Build history of the part. All positions in model axes, mm. Face numbers are marked on the shaded views. A direction names the side the tool comes from. Coordinates: 2 decimals unless noted, no trailing zeros. Order: outer loops, then holes, each group sorted by start corner. A loop starts at its lowest first (then second) coordinate and runs counter-clockwise, first axis right, second up. Notation, with made-up numbers: (-38, -17.75) - (-19, -17.75) arc R23 cw to (-19, 8.25) - close; hole circle Ø3 at (-29.75, 76.5). An arc over 180 degrees is marked (long way). One line per item, written item: value.
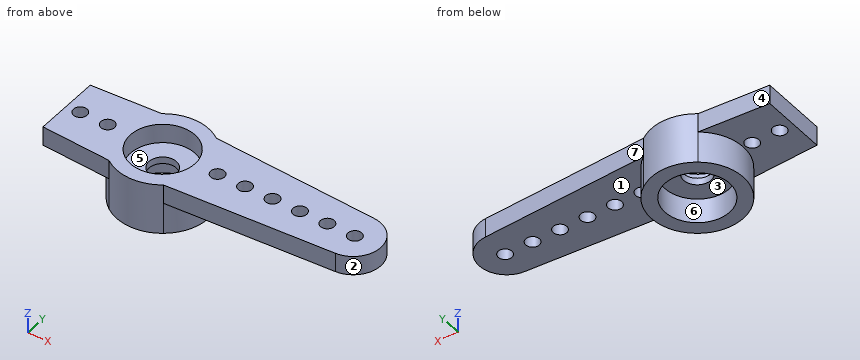
from build123d import *

# Parameters (mm, degrees)
F0_R     = 2.35
F0_R_2   = 0.5
F1_DEPTH = 1.4
F2_R     = 2.35
F2_R_2   = 1
F3_DEPTH = 2.3
F4_R     = 2.35
F4_R_2   = 1
F5_DEPTH = 1.8


with BuildPart() as f1:
    # F0 (on Top) → F1 (new body)
    with BuildSketch(Plane.XY):
        with BuildLine():
            ThreePointArc((1.9830532015, -2.7), (2.9887897404, -1.5131542841), (3.35, 0))
            ThreePointArc((3.35, 0), (2.9887897404, 1.5131542841), (1.9830532015, 2.7))
            ThreePointArc((1.9830532015, 2.7), (0, 3.35), (-1.9830532015, 2.7))
            ThreePointArc((-1.9830532015, 2.7), (-3.35, 0), (-1.9830532015, -2.7))
            ThreePointArc((-1.9830532015, -2.7), (0, -3.35), (1.9830532015, -2.7))
        make_face()
        Circle(F0_R, mode=Mode.SUBTRACT)
        with BuildLine():
            ThreePointArc((1.9830532015, 2.7), (2.9887897404, 1.5131542841), (3.35, 0))
            ThreePointArc((3.35, 0), (2.9887897404, -1.5131542841), (1.9830532015, -2.7))
            Line((1.9830532015, -2.7), (14, -2))
            ThreePointArc((14, -2), (15.886888175, 0), (14, 2))
            Line((14, 2), (1.9830532015, 2.7))
        make_face()
        with Locations((4, 0)):
            Circle(F0_R_2, mode=Mode.SUBTRACT)
        with Locations((6, 0)):
            Circle(F0_R_2, mode=Mode.SUBTRACT)
        with Locations((8, 0)):
            Circle(F0_R_2, mode=Mode.SUBTRACT)
        with Locations((10, 0)):
            Circle(F0_R_2, mode=Mode.SUBTRACT)
        with Locations((12, 0)):
            Circle(F0_R_2, mode=Mode.SUBTRACT)
        with Locations((14, 0)):
            Circle(F0_R_2, mode=Mode.SUBTRACT)
        with BuildLine():
            ThreePointArc((-1.9830532015, -2.7), (-3.35, 0), (-1.9830532015, 2.7))
            Line((-1.9830532015, 2.7), (-6.9970610693, 2.4079286805))
            Line((-6.9970610693, 2.4079286805), (-6.9970610693, -2.4079286805))
            Line((-6.9970610693, -2.4079286805), (-1.9830532015, -2.7))
        make_face()
        with Locations((-6, 0)):
            Circle(F0_R_2, mode=Mode.SUBTRACT)
        with Locations((-4, 0)):
            Circle(F0_R_2, mode=Mode.SUBTRACT)
    extrude(amount=F1_DEPTH)

    # F2 (on face) → F3 (join)
    with BuildSketch(Plane(origin=(0, 0, 0), x_dir=(1, 0, 0), z_dir=(0, 0, -1))):
        with BuildLine():
            ThreePointArc((1.9830532015, -2.7), (2.9887897404, -1.5131542841), (3.35, 0))
            ThreePointArc((3.35, 0), (2.9887897404, 1.5131542841), (1.9830532015, 2.7))
            ThreePointArc((1.9830532015, 2.7), (0, 3.35), (-1.9830532015, 2.7))
            ThreePointArc((-1.9830532015, 2.7), (-3.35, 0), (-1.9830532015, -2.7))
            ThreePointArc((-1.9830532015, -2.7), (0, -3.35), (1.9830532015, -2.7))
        make_face()
        Circle(F2_R, mode=Mode.SUBTRACT)
        Circle(F2_R)
        Circle(F2_R_2, mode=Mode.SUBTRACT)
    extrude(amount=F3_DEPTH)

    # F4 (on face) → F5 (cut)
    with BuildSketch(Plane(origin=(0, 0, -2.3), x_dir=(1, 0, 0), z_dir=(0, 0, -1))):
        Circle(F4_R)
        Circle(F4_R_2, mode=Mode.SUBTRACT)
    extrude(amount=-F5_DEPTH, mode=Mode.SUBTRACT)


solid = f1.part
1. 3-axis set-ups, long thin cutter, end or side, ignore diameter. For the marked faces 5, 6 and 7: which of +Z, -Z, +X, -X, +Y, -Y reach the whole face in a straight line?
Values found:
face 5: +Z
face 6: -Z
face 7: +Z, -Z, +X, +Y
2. Band-saw the part on A-A, the plane z = 0.35. Count the separate pieces of the cut face and the enclosed holes in it, and give its area (3 significant figures).
Values found:
separate pieces: 1
enclosed holes: 9
area: 89.2 mm2
3. Probe line 1 along Y through (x, z) = (8, 0.7); line 2 along X through (y, z) = (0, -1.5); line 3 along Z through (x, y) = (-3.5, -1.5). List the from-to ranges inside material, lowest first.
Values found:
line 1: y = -2.35 to -0.5, 0.5 to 2.35
line 2: x = -3.35 to -2.35, 2.35 to 3.35
line 3: z = 0 to 1.4
4. Band-saw the part on C-C, the plane y = 1.5. Give the cut face in (x, z).
Values found:
outline: (-7, 0) - (-3, 0) - (-3, -2.3) - (-1.81, -2.3) - (-1.81, -0.5) - (1.81, -0.5) - (1.81, -2.3) - (3, -2.3) - (3, 0) - (15.21, 0) - (15.21, 1.4) - (1.81, 1.4) - (1.81, 0) - (-1.81, 0) - (-1.81, 1.4) - (-7, 1.4) - close
5. Band-saw the part on B-B, the plane x = 12. Give the cut face in (y, z), and give its area (3 significant figures).
Values found:
outline: (-2.12, 0) - (-0.5, 0) - (-0.5, 1.4) - (-2.12, 1.4) - close; (0.5, 0) - (2.12, 0) - (2.12, 1.4) - (0.5, 1.4) - close
area: 4.53 mm2
6. Band-saw the part on D-D, the plane z = -1.55. Give the cut face in (x, y).
Values found:
outline: circle Ø6.7 at (0, 0); hole circle Ø4.7 at (0, 0)
7. Flat gauge pins, fed straight in: P1, Ø1.6, axis at x = 7.5, y = 1, coming from the -Z side; P2, Ø1.4, axis at x = -1, y = -0.5, coming from the +Z side; P3, Ø1.5, axis at y = -1.5, z = -1, coming from the +X side; P4, Ø1.6, axis at x = 0, y = 0, coming from the -Z side. Where does each tip first touch, or does it go through?
Values found:
P1: stops at z = 0
P2: stops at z = 0
P3: stops at x = 3.26
P4: passes through
8. Two-plate mould, pull along Y, no slides. Class the marked faces 1, 2, 3 and 4: pulls with the +Y half, pulls with the -Y half, needs draft (parallel to the pull), parting line crosses it, or undercut.
Values found:
face 1: needs draft
face 2: parting line crosses it
face 3: undercut
face 4: pulls with the +Y half
